from build123d import *

# Parameters (mm, degrees)
PAD003003002_DEPTH = 42.25
SKETCH009_W        = 52
SKETCH009_H        = 3
PAD003003003_DEPTH = 1.5
SKETCH010_W        = 43.5
SKETCH010_H        = 78.5
POCKET002_DEPTH    = 2


with BuildPart() as part:
    # Sketch008 → Pad003003002 (new body, symmetric)
    with BuildSketch(Plane.YZ):
        Polygon((22.75, 28), (-22.75, 28), (-22.75, 27), (-23.75, 26), (-23.75, 25), (23.75, 25), (23.75, 26), (22.75, 27), align=None)
    extrude(amount=PAD003003002_DEPTH, both=True)

    # Sketch009 → Pad003003003 (new body)
    with BuildSketch(Plane.YZ.offset(42.25)):
        with Locations((0, 26.5)):
            Rectangle(SKETCH009_W, SKETCH009_H)
    extrude(amount=PAD003003003_DEPTH)

    # Sketch010 → Pocket002 (cut)
    with BuildSketch(Plane.YX.offset(-25)):
        with Locations((0, 3)):
            Rectangle(SKETCH010_W, SKETCH010_H)
    extrude(amount=-POCKET002_DEPTH, mode=Mode.SUBTRACT)


solid = part.part
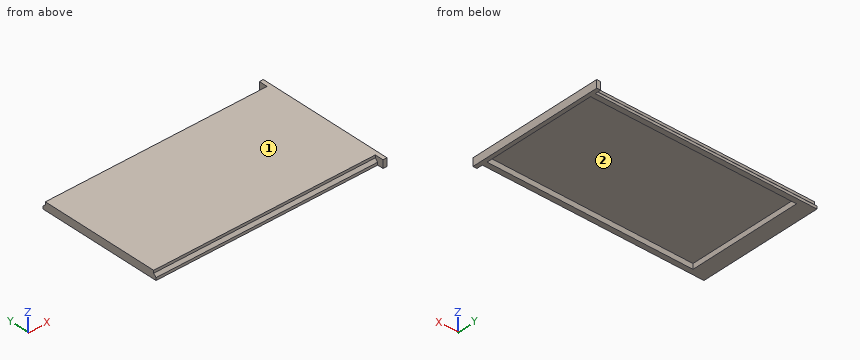
For this review, take the finished solid that the model builds, in its own axes (mm). Face numbers are marked on the shaded views. Round coordinates to 2 decimals unless told otherwise and drop trailing zeros. Write each loop counter-clockwise with the first axis right and the second up, starting at its lowest first coordinate (ties: lowest second). Pieces come first, ordered by that corner, then holes. Notation, with made-up numbers: (-39.5, -15) -> (-13.5, -15) arc R27 cw to (-13.5, 23) -> close; hole circle Ø9 at (-26, 58). An arc over 180 degrees is marked (long way). Put each result on its own line as item: value.
Q1. To check wall thickness, follow L1, parallel to X at y = -1, z = 26.15; L2, parallel to Y at x = -5.5, z = 25.5; L3, parallel to Z at x = -27.5, y = -13. State the ranges of each line that lie inside material, in increasing order. Write a range as [from, to].
Determined:
L1: x = [-42.25, -36.25], [42.25, 43.75]
L2: y = [-23.75, -21.75], [21.75, 23.75]
L3: z = [27, 28]
Q2. Consider section B-B on z = 25.5. State the section outline as (x, y) points, and give its area (3 significant figures).
Determined:
outline: (-42.25, -23.75) -> (42.25, -23.75) -> (42.25, -26) -> (43.75, -26) -> (43.75, 26) -> (42.25, 26) -> (42.25, 23.75) -> (-42.25, 23.75) -> close; hole (-36.25, -21.75) -> (42.25, -21.75) -> (42.25, 21.75) -> (-36.25, 21.75) -> close
area: 677 mm^2
Q3. Consider section C-C on y = 0. State the section outline as (x, z) points.
Determined:
outline: (-42.25, 25) -> (-36.25, 25) -> (-36.25, 27) -> (42.25, 27) -> (42.25, 25) -> (43.75, 25) -> (43.75, 28) -> (-42.25, 28) -> close
Q4. Clearance check with flat-ended pins moving along their axes: pin 1 Ø0.8 at (x, z) = (9, 25.5) entering from -Y; pin 2 Ø1 at (x, z) = (21.5, 26) entering from +Y; pin 3 Ø1.1 at (x, z) = (-11.5, 27.5) entering from -Y. State where each tip first meets the part, or that it passes through.
Determined:
pin 1: stops at y = -23.75
pin 2: stops at y = 23.75
pin 3: stops at y = -22.8
Q5. The part is to be moulded in two halves that separate along X. For the marked faces 1 and 2, say which applies: released by +X, released by -X, zero draft, split by the parting line, or undercut.
Determined:
face 1: zero draft
face 2: undercut
Q6. Consider section A-A on x = 31. State the section outline as (y, z) points, and give its area (3 significant figures).
Determined:
outline: (-23.75, 25) -> (-21.75, 25) -> (-21.75, 27) -> (21.75, 27) -> (21.75, 25) -> (23.75, 25) -> (23.75, 26) -> (22.75, 27) -> (22.75, 28) -> (-22.75, 28) -> (-22.75, 27) -> (-23.75, 26) -> close
area: 52.5 mm^2
